Input: dimensioned drawing with shaded views. Units: mm. Origin: part minimum x, y, z. A direction names the side the tool comes from. Coordinates: 2 decimals unless noted, no trailing zeros. Loops run counter-clockwise (first coordinate to the right, second up) from the corner with the lowest first, then second, coordinate; pieces in that order, holes last.
Item 1: Section query A-A, the plane z = 10. Return the cut outline in (x, y), then the cut area to 3 significant figures.
Item 2: Section query D-D, the plane x = 6.75. Return the cut outline in (y, z), then the cut area to 3 significant figures.
Item 3: Pull-direction query (Y, two-part tool) for the marked faces 1, 2 and 3; classes: +Y half, -Y half, draft (parallel to the pull), parting line (faces both ways), or undercut.
Item 4: Pin query (flat end, axial travel): pin 1 Ø6 at (y, z) = (10, 10.5) entering from +X. Return the tip coordinate at first contact, or that it passes through.
Item 5: Line query: probe 1 along Y at (x, z) = (1.65, 10); probe 2 along Y at (x, z) = (21.25, 12); probe 3 along X at (y, z) = (14.5, 4.5). Output: solid intervals per line, ascending.
Item 6: Reachability of the marked faces 4 and 5 from +Z, -Z, +X, -X, +Y, -Y: full face, straight path, thin tool, end or side. Return the list, or none.
Item 7: Section query C-C, the plane z = 17.5. Return the cut outline in (x, y).
Item 8: Section query B-B, the plane x = 3. Return the cut outline in (y, z).
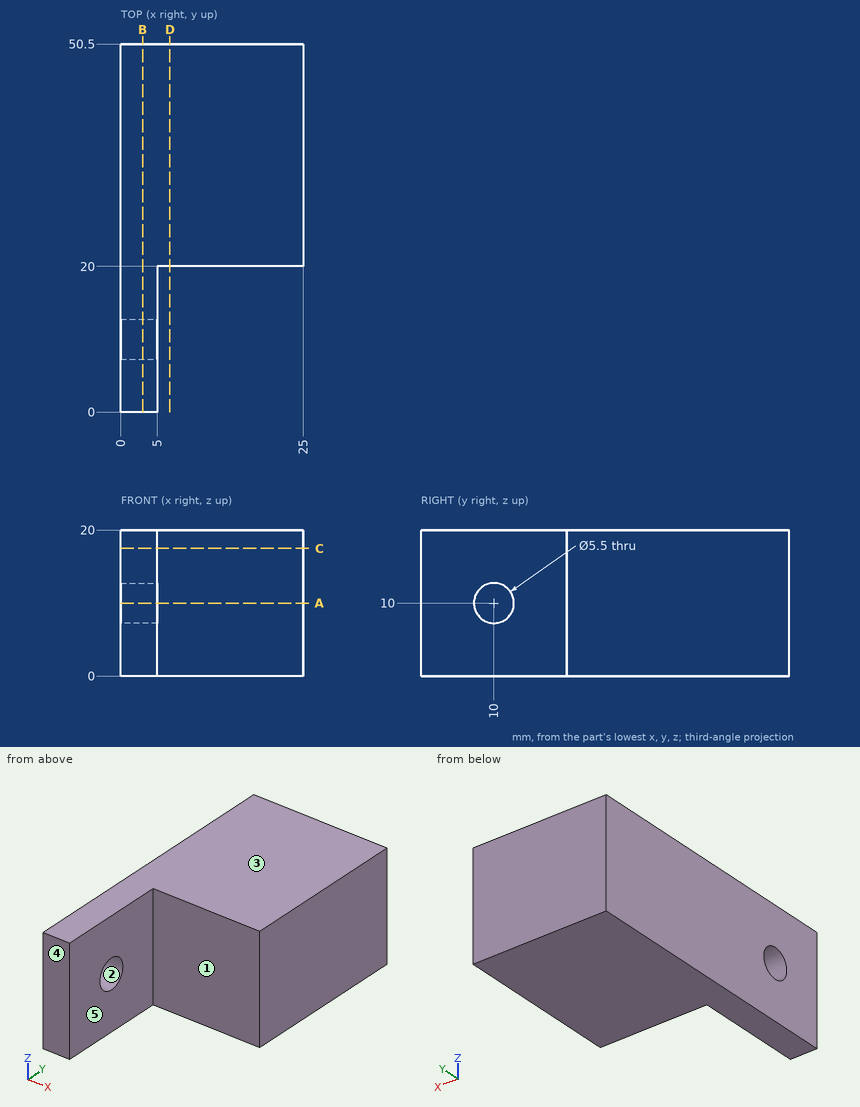
Verdict:
1. outline: (0, 0) - (5, 0) - (5, 7.25) - (0, 7.25) - close; (0, 12.75) - (5, 12.75) - (5, 20) - (25, 20) - (25, 50.5) - (0, 50.5) - close
1. area: 835 mm2
2. outline: (20, 0) - (50.5, 0) - (50.5, 20) - (20, 20) - close
2. area: 610 mm2
3. face 1: -Y half
3. face 2: undercut
3. face 3: draft
4. pin 1: stops at x = 5
5. probe 1: y = 0 to 7.25, 12.75 to 50.5
5. probe 2: y = 20 to 50.5
5. probe 3: x = 0 to 5
6. face 4: +Z, -Z, +X, -X, -Y
6. face 5: +Z, -Z, +X, -Y
7. outline: (0, 0) - (5, 0) - (5, 20) - (25, 20) - (25, 50.5) - (0, 50.5) - close
8. outline: (0, 0) - (50.5, 0) - (50.5, 20) - (0, 20) - close; hole circle Ø5.5 at (10, 10)
